Work out the finished part from the listing and answer in its coordinate system (mm). A direction names the side the tool comes from. Round coordinates to 2 decimals unless told otherwise and drop trailing zeros. Write each loop counter-clockwise with the first axis right and the second up, starting at its lowest first coordinate (ties: lowest second). Pieces come first, ordered by that corner, then holes. Notation, with made-up numbers: (84, 0.25) - (142, 0.25) arc R23 ccw to (142, 11.25) - close; hole circle Ø8 at (22.25, -28.75). An arc over 180 degrees is marked (long way). Answer as a JSON object with one key per item and string values.
```python
from build123d import *

# Parameters (mm, degrees)
F0_R     = 35
F1_DEPTH = 23
F2_T     = -1
F3_R     = 2


# Not quite as in the source:
# - a feature of the source that left no trace in its solid (it failed there, or was rolled back) is left out


with BuildPart() as f1:
    # F0 (on Front) → F1 (new body)
    with BuildSketch(Plane.XZ):
        Circle(F0_R)
    extrude(amount=F1_DEPTH)

    # F2
    f2_openings = [f1.faces().sort_by_distance(p)[0] for p in [
        (0, 0, 0),
    ]]
    offset(amount=F2_T, openings=f2_openings)

    # F3
    f3_edges = [f1.edges().sort_by_distance(p)[0] for p in [
        (-35, -23, 0),
    ]]
    fillet(f3_edges, radius=F3_R)


solid = f1.part
```
Item 1: A cutting plane is placed at C-C (y = -16). Write down the section's boundary in (x, z), and give its area (3 significant figures).
Results found:
{"outline": "circle Ø70 at (0, 0); hole circle Ø68 at (0, 0)", "area": "217 mm²"}
Item 2: A cutting plane is placed at A-A (z = 0). Write down the section's boundary in (x, y).
Results found:
{"outline": "(-35, -21) arc R2 ccw to (-33, -23) - (33, -23) arc R2 ccw to (35, -21) - (35, 0) - (34, 0) - (34, -22) - (-34, -22) - (-34, 0) - (-35, 0) - close"}
Item 3: A cutting plane is placed at B-B (x = 0). Write down the section's boundary in (y, z).
Results found:
{"outline": "(-23, -33) arc R2 ccw to (-21, -35) - (0, -35) - (0, -34) - (-22, -34) - (-22, 34) - (0, 34) - (0, 35) - (-21, 35) arc R2 ccw to (-23, 33) - close"}
Item 4: Consider line 1 along Z through (x, y) = (0, -13.25); line 2 along Y through (x, z) = (18, -1.5); line 3 along X through (y, z) = (-4, 16). Determine where each line is inside the solid, lowest interval first.
Results found:
{"line 1": "-35 to -34, 34 to 35", "line 2": "-23 to -22", "line 3": "-31.13 to -30, 30 to 31.13"}
Item 5: Each of these flat-tipped pins is pushed along its axis until it touches: P1, Ø12, axis at x = 27.5, y = -17.5, coming from the -Z side; P2, Ø4, axis at x = 3.5, z = 20, coming from the +Y side; P3, Ø5, axis at x = 6.5, y = -13, coming from the -Z side. Where does it stop, or does it pass through?
Results found:
{"P1": "z = -27.62", "P2": "y = -22", "P3": "z = -34.77"}
Item 6: For faces 1 (the flat face through (0, -22, 0)), 2 (the flat face through (-5, 0, 34)), determine the directions among +Z, -Z, +X, -X, +Y, -Y from which every point of the face is accessible in a straight line to the end or side of a thin tool.
Results found:
{"face 1": "+Y", "face 2": "+Z, -Z, +X, -X, +Y"}
Item 7: Determine the mould class of faces 3 (the cylindrical face through (18.28, -10.85, 28.67)), 4 (the flat face through (0, -23, 0)), 5 (the cylindrical face through (-28, -10, -21)) for opening direction X: pulls with the +X half, pulls with the -X half, needs draft (parallel to the pull), parting line crosses it, or undercut.
Results found:
{"face 3": "undercut", "face 4": "needs draft", "face 5": "parting line crosses it"}
